from build123d import *

# Parameters (mm, degrees)
SWEEP1_PROFILE_R   = 5
SWEEP4_PROFILE_R   = 5
SWEEP5_PROFILE_R   = 5
SPLIT1_START       = 5
SPLIT1_OUTLINE_W   = 10
SPLIT1_OUTLINE_H   = 12
SPLIT1_DEPTH       = 9.304379119
SKETCH37_R         = 3.5
CUT_EXTRUDE1_DEPTH = 49
SKETCH38_R         = 3.5
CUT_EXTRUDE2_DEPTH = 132
SKETCH39_R         = 3.5
CUT_EXTRUDE3_DEPTH = 132


# Read off the part's stored shape, not the designer's step: Split1
with BuildPart() as part:
    # Sweep1: sweep along a path in Sketch1
    with BuildLine(Plane(origin=(0, 0, 0), x_dir=(1, 0, 0), z_dir=(0, 1, 0))) as sweep1_path:
        Line((-62.917795488, 168.645637391), (0, 0))
        Line((0, 0), (62.917795488, 168.645637391))
    # Sweep1 profile (on start of the path) → Sweep1 (sweep)
    with BuildSketch(Plane(origin=(-62.917795488, 0, -168.645637391), x_dir=(0.936920207726199, 0, -0.349543308267082), z_dir=(0.349543308267082, 0, 0.936920207726199))):
        Circle(SWEEP1_PROFILE_R)
    sweep(path=sweep1_path.line, transition=Transition.RIGHT)

    # Sweep4: sweep along a path in Sketch1<7>
    with BuildLine(Plane(origin=(0, 0, 0), x_dir=(1, 0, 0), z_dir=(0, 1, 0))) as sweep4_path:
        Line((0, 40), (0, -5))
    # Sweep4 profile (on start of the path) → Sweep4 (sweep)
    with BuildSketch(Plane.XY.offset(-40)):
        Circle(SWEEP4_PROFILE_R)
    sweep(path=sweep4_path.line)

    # Sweep5: sweep along a path in Sketch1<8>
    with BuildLine(Plane(origin=(0, 0, 0), x_dir=(1, 0, 0), z_dir=(0, 1, 0))) as sweep5_path:
        Line((48.5, 130), (-48.5, 130))
    # Sweep5 profile (on start of the path) → Sweep5 (sweep)
    with BuildSketch(Plane(origin=(48.5, 0, -130), x_dir=(0, 0, -1), z_dir=(-1, 0, 0))):
        Circle(SWEEP5_PROFILE_R)
    sweep(path=sweep5_path.line)

    # Split1 outline → Split1 (cut)
    with BuildSketch(Plane.XY.offset(SPLIT1_START)):
        Rectangle(SPLIT1_OUTLINE_W, SPLIT1_OUTLINE_H)
    extrude(amount=SPLIT1_DEPTH, mode=Mode.SUBTRACT)

    # Sketch37 → Cut-Extrude1 (cut)
    with BuildSketch(Plane.XY.offset(5)):
        Circle(SKETCH37_R)
    extrude(amount=-CUT_EXTRUDE1_DEPTH, mode=Mode.SUBTRACT)

    # Sketch38 → Cut-Extrude2 (cut)
    with BuildSketch(Plane(origin=(-62.917795488, 0, -168.645637391), x_dir=(-0.9369202077261991, 0, 0.34954330826708174), z_dir=(-0.34954330826708174, 0, -0.9369202077261991))):
        Circle(SKETCH38_R)
    extrude(amount=-CUT_EXTRUDE2_DEPTH, mode=Mode.SUBTRACT)

    # Sketch39 → Cut-Extrude3 (cut)
    with BuildSketch(Plane(origin=(62.917795488, 0, -168.645637391), x_dir=(-0.9369202077261989, 0, -0.3495433082670822), z_dir=(0.3495433082670822, 0, -0.9369202077261989))):
        Circle(SKETCH39_R)
    extrude(amount=-CUT_EXTRUDE3_DEPTH, mode=Mode.SUBTRACT)


solid = part.part
Model file for the job. Use its own axes, mm. A direction names the side the tool comes from. Give positions to 0.01 mm unless a question says otherwise; leave off trailing zeros. Order: outer loops, then holes, each group sorted by start corner. A loop starts at its lowest first (then second) coordinate and runs counter-clockwise, first axis right, second up. Notation, with made-up numbers: (-28, -15.5) - (2, -15.5) arc R26 cw to (2, 12.5) - close; hole circle Ø5 at (83, 29). An arc over 180 degrees is marked (long way). Write item = value, one per line. Start each with the question number.
1. Probe line 1 along Y through (x, z) = (0, -3); line 2 along X through (y, z) = (-3, -106.5); line 3 along X through (y, z) = (1, -75). List the from-to ranges inside material, lowest first.
2. Two-plate mould, pull along Z, no slides. Class faces 5 (the cylindrical face through (3.233, -1.341, -17.185)), 6 (the flat face through (-60.9, -3.3, -169.4)), 7 (the flat face through (16.824, 0.049, -44.955)), 8 (the flat face through (2.2, -3.3, 5)): pulls with the +Z half, pulls with the -Z half, needs draft (parallel to the pull), parting line crosses it, or undercut.
3. Which spindle directions (+Z, -Z, +X, -X, +Y, -Y) get a long thin tool onto all of the face, cutting with end or side? Do faces 1 (the flat face through (60.9, -3.3, -169.4)), 2 (the flat face through (2.2, -3.3, -40)), 3 (the flat face through (-16.7, 0, -45)), 4 (the cylindrical face through (4.77, 1.5, 2.53)). Say none if no direction does.
4. Drop flat-ended pins along their axis: P1, Ø3, axis at x = 0.5, y = -2, coming from the -Z side; P2, Ø5, axis at y = -3, z = -117, coming from the +X side; P3, Ø2, axis at y = -2, z = -128, coming from the -X side. Give the stop position or say it passes through.
5. Cut at A-A, the plane y = -2. List the corners of the cut face in (x, z).
6. Cut at B-B, the plane z = -75. State how many separate pieces and enclosed holes the cut face has, and give its area (3 significant figures).
Taken from the geometry:
q1.line_1 = -5 to -3.5, 3.5 to 5
q1.line_2 = -44 to -41.66, -37.81 to -35.46, 35.46 to 37.81, 41.66 to 44
q1.line_3 = -33.21 to -31.56, -24.4 to -22.75, 22.75 to 24.4, 31.56 to 33.21
q2.face_5 = needs draft
q2.face_6 = pulls with the -Z half
q2.face_7 = undercut
q2.face_8 = pulls with the +Z half
q3.face_1 = -Z, +X, +Y, -Y
q3.face_2 = +Y, -Y
q3.face_3 = none
q3.face_4 = +Z
q4.P1 = -134.97
q4.P2 = 49.49
q4.P3 = -53.18
q5.outline = (-67.21, -167.04) - (-65.61, -167.64) - (-19.47, -43.97) - (-14.09, -45.98) - (-60.23, -169.65) - (-58.62, -170.25) - (-45.32, -134.58) - (45.32, -134.58) - (58.62, -170.25) - (60.23, -169.65) - (14.09, -45.98) - (19.47, -43.97) - (65.61, -167.64) - (67.21, -167.04) - (4.58, 0.83) - (4.58, 5) - (2.87, 5) - (2.87, -40) - (4.58, -40) - (4.58, -25.39) - (41.9, -125.42) - (-41.9, -125.42) - (-4.58, -25.39) - (-4.58, -40) - (-2.87, -40) - (-2.87, 5) - (-4.58, 5) - (-4.58, 0.83) - close
q6.separate_pieces = 2
q6.enclosed_holes = 2
q6.area = 85.5 mm²
